```python
from build123d import *

# Parameters (mm, degrees)
F0_R     = 31
F0_R_2   = 21.5
F1_DEPTH = 25
F2_W     = 8.098436
F2_H     = 15.167526
F3_DEPTH = 25
F4_T     = -2.5


with BuildPart() as f1:
    # F0 (on Top) → F1 (new body)
    with BuildSketch(Plane.XY):
        Circle(F0_R)
        Circle(F0_R_2, mode=Mode.SUBTRACT)
    extrude(amount=F1_DEPTH)

    # F2 (on face) → F3 (cut)
    with BuildSketch(Plane.XY.offset(25)):
        with Locations((0, 25.295008)):
            Rectangle(F2_W, F2_H)
    extrude(amount=-F3_DEPTH, mode=Mode.SUBTRACT)

    # F4
    f4_openings = [f1.faces().sort_by_distance(p)[0] for p in [
        (0, -30.125064, 0),
        (-4.924154, 25.92483, 25),
    ]]
    offset(amount=F4_T, openings=f4_openings)


solid = f1.part
```
Source: CAD feature listing. Evaluate the final solid. Frame: model axes, mm. A direction names the side the tool comes from. Round coordinates to 2 decimals unless told otherwise and drop trailing zeros. Loops run counter-clockwise (first coordinate to the right, second up) from the corner with the lowest first, then second, coordinate; pieces in that order, holes last.
1. Contact query for flat-ended pins moving along their axis: pin 1 (12 mm diameter, centred on x = -10, z = 16.5, fed in from -Y); pin 2 (12 mm diameter, centred on x = 11.5, z = 14, fed in from -Y); pin 3 (8 mm diameter, centred on x = -8.5, z = 19, fed in from +Y). Output: stop coordinate, or through.
2. Access query for faces 1 (the flat face through (-4.049, 26, 13)), 2 (the flat face through (-11.6, -18.3, 0)), 3 (the flat face through (-6.549, 25, 13)). Directions: +Z, -Z, +X, -X, +Y, -Y. A direction counts if a zero-diameter tool reaches every point of the face in a straight line with its end or side. Return the directions, or none.
3. Ray query, L1, parallel to X at y = 0, z = 13.5; L2, parallel to Y at x = 0, z = 19.5; L3, parallel to Y at x = -11, z = 15. Return the intervals inside material, ascending.
4. Section query A-A on y = 0. Output: boundary loops of the cut face in (x, z).
5. Mould query, pull axis Y, two halves, no side actions, for faces 4 (the cylindrical face through (-1.161, -28.476, 12.325)), 5 (the cylindrical face through (-1.306, -30.972, 12.325)), 6 (the flat face through (-11.6, -18.3, 25)). Classes: released by +Y, released by -Y, zero draft, split by the parting line, or undercut.
6. Section query C-C on z = 19.5. Output: boundary loops of the cut face in (x, y), and give its area (3 significant figures).
7. Section query D-D on y = -25.5. Output: boundary loops of the cut face in (x, z), and give its area (3 significant figures).
8. Section query B-B on x = 0. Output: boundary loops of the cut face in (y, z), and give its area (3 significant figures).
Answers below:
1. pin 1: stops at y = -30.74
1. pin 2: stops at y = -30.51
1. pin 3: stops at y = 30.67
2. face 1: +Z, -Z, +Y
2. face 2: -Z, +X, -X, +Y, -Y
2. face 3: +Z, -Z
3. L1: x = -31 to -28.5, -24 to -21.5, 21.5 to 24, 28.5 to 31
3. L2: y = -31 to -28.5, -24 to -21.5
3. L3: y = -28.98 to -26.29, -21.33 to -18.47, 18.47 to 21.33, 26.29 to 28.98
4. outline: (-31, 0) - (-28.5, 0) - (-28.5, 25) - (-31, 25) - close; (-24, 0) - (-21.5, 0) - (-21.5, 25) - (-24, 25) - close; (21.5, 0) - (24, 0) - (24, 25) - (21.5, 25) - close; (28.5, 0) - (31, 0) - (31, 25) - (28.5, 25) - close
5. face 4: undercut
5. face 5: split by the parting line
5. face 6: zero draft
6. outline: (-4.05, 21.12) - (-4.05, 30.73) arc R31 ccw (long way) to (4.05, 30.73) - (4.05, 21.12) arc R21.5 cw (long way) to start; hole (-6.55, 23.09) - (-6.55, 27.74) arc R28.5 ccw (long way) to (6.55, 27.74) - (6.55, 23.09) arc R24 cw (long way) to start
6. area: 807 mm2
7. outline: (-17.63, 0) - (-12.73, 0) - (-12.73, 25) - (-17.63, 25) - close; (12.73, 0) - (17.63, 0) - (17.63, 25) - (12.73, 25) - close
7. area: 245 mm2
8. outline: (-31, 0) - (-28.5, 0) - (-28.5, 25) - (-31, 25) - close; (-24, 0) - (-21.5, 0) - (-21.5, 25) - (-24, 25) - close
8. area: 125 mm2
